from build123d import *

# Parameters (mm, degrees)
PAD_DEPTH       = 3
SKETCH001_R     = 1
POCKET_DEPTH    = 3
SKETCH002_W     = 26
SKETCH002_H     = 22
POCKET001_DEPTH = 0.5


with BuildPart() as part:
    # Sketch → Pad (new body)
    with BuildSketch(Plane.XY):
        Polygon((15, -15), (15, 15), (-15, 15), (-15, -15), (-9, -15), (-9, 5), (9, 5), (9, -15), align=None)
    extrude(amount=PAD_DEPTH)

    # Sketch001 (on Face10 of Pad) → Pocket (cut)
    with BuildSketch(Plane.XY.offset(3)):
        with Locations((-12, 12)):
            Circle(SKETCH001_R)
        with Locations((12, 12)):
            Circle(SKETCH001_R)
    extrude(amount=-POCKET_DEPTH, mode=Mode.SUBTRACT)

    # Sketch002 (on Face5 of Pocket) → Pocket001 (cut)
    with BuildSketch(Plane.XY.offset(3)):
        with Locations((0, -3)):
            Rectangle(SKETCH002_W, SKETCH002_H)
    extrude(amount=-POCKET001_DEPTH, mode=Mode.SUBTRACT)


solid = part.part
Here's how the part is built. I have some questions about the finished solid (model axes, mm). A direction names the side the tool comes from. Coordinates: 2 decimals unless noted, no trailing zeros. Write each loop counter-clockwise with the first axis right and the second up, starting at its lowest first coordinate (ties: lowest second). Pieces come first, ordered by that corner, then holes.
1) If we section it at B-B (z = 1.2): List the corners of the cut face in (x, y) for me.
Filled in:
outline: (-15, -15) - (-9, -15) - (-9, 5) - (9, 5) - (9, -15) - (15, -15) - (15, 15) - (-15, 15) - close; hole circle Ø2 at (-12, 12); hole circle Ø2 at (12, 12)
2) If we section it at A-A (y = 12): List the corners of the cut face in (x, z) for me.
Filled in:
outline: (-15, 0) - (-13, 0) - (-13, 3) - (-15, 3) - close; (-11, 0) - (11, 0) - (11, 3) - (-11, 3) - close; (13, 0) - (15, 0) - (15, 3) - (13, 3) - close
3) Thinking about a two-plate mould opening in Y: for faces 4 (the face through (-12, -15, 1)), 5 (the face through (-9, -5, 1)), 6 (the face through (11.2, 11.4, 1.5)), which applies, +Y half, -Y half, draft (parallel to the pull), parting line (faces both ways), or undercut?
Filled in:
face 4: -Y half
face 5: draft
face 6: undercut
4) If we section it at D-D (y = -13): List the corners of the cut face in (x, z) for me, plus the area to 3 significant figures.
Filled in:
outline: (-15, 0) - (-9, 0) - (-9, 2.5) - (-13, 2.5) - (-13, 3) - (-15, 3) - close; (9, 0) - (15, 0) - (15, 3) - (13, 3) - (13, 2.5) - (9, 2.5) - close
area: 32.0 mm2
5) Which directions (+Z, -Z, +X, -X, +Y, -Y) give clear straight access to the entire face, cutting with the end or side of a thin tool? Please do faces 1 (the face through (9, -5, 1)), 2 (the face through (-1, 5.2, 2.5)), 3 (the face through (12, -15, 1)).
Filled in:
face 1: +Z, -Z, -Y
face 2: +Z
face 3: +Z, -Z, +X, -X, -Y
6) If I drill on line 1 (X direction, y = -13, z = 0.25); line 2 (Y direction, x = -12, z = 0.9); line 3 (Z direction, x = -9.25, y = -6), over which ranges is the centre line in solid material (lowest first)?
Filled in:
line 1: x = -15 to -9, 9 to 15
line 2: y = -15 to 11, 13 to 15
line 3: z = 0 to 2.5
7) I'm going to push flat-ended pins straight in: pin 1 (0.8 mm diameter, centred on x = -3.5, z = 0.5, fed in from -Y); pin 2 (11 mm diameter, centred on x = -5.5, y = 0.5, fed in from +Z). Where does each tip first touch, or does it pass through?
Filled in:
pin 1: stops at y = 5
pin 2: stops at z = 2.5
8) If we section it at C-C (x = -12): List the corners of the cut face in (y, z) for me.
Filled in:
outline: (-15, 0) - (11, 0) - (11, 3) - (8, 3) - (8, 2.5) - (-14, 2.5) - (-14, 3) - (-15, 3) - close; (13, 0) - (15, 0) - (15, 3) - (13, 3) - close
